Could you check a few things on this model? Use its own coordinates, in mm. Face numbers are marked on the shaded views. A direction names the side the tool comes from. Coordinates: 2 decimals unless noted, no trailing zeros. Order: outer loops, then holes, each group sorted by start corner. A loop starts at its lowest first (then second) coordinate and runs counter-clockwise, first axis right, second up. Notation, with made-up numbers: (-15.75, -1) -> (37.25, -1) arc R31 cw to (37.25, 26) -> close; hole circle Ø3 at (-38, 25.25). An arc over 180 degrees is marked (long way). Put each result on its own line as item: value. Start each with the question number.
Q1. If we section it at D-D (y = 30.5): Please give me the cut outline in (x, z).
Q2. We'd pull the mould along X, two halves only. Please class the marked faces 1, 2 and 3: +X half, -X half, draft (parallel to the pull), parting line (faces both ways), or undercut.
Q3. If we section it at B-B (y = 6): Please give me the cut outline in (x, z).
Q4. Please list where these lines run through material, in increasing order: line 1 along Z through (x, y) = (9, 22.5); line 2 along Y through (x, z) = (-1.5, 10.75); line 3 along X through (y, z) = (25.5, -3.25).
Q5. Will these pins go through, and if not, where does the flat tip stop? pin 1 (5 mm diameter, centred on x = -5.5, z = 4, fed in from +Y); pin 2 (11 mm diameter, centred on y = 20, z = -2.5, fed in from -X); pin 3 (3.5 mm diameter, centred on y = 30.5, z = -13, fed in from -X).
Q6. For the marked faces 4, 5 and 6, which set-ups out of +Z, -Z, +X, -X, +Y, -Y let a thin tool reach every point of the face, with its end or its side?
Q7. If we section it at A-A (z = 0): Please give me the cut outline in (x, y).
Q8. If we section it at C-C (x = 6.5): Please give me the cut outline in (y, z), and give its area (3 significant figures).
from build123d import *

# Parameters (mm, degrees)
SKETCH1_W               = 35
SKETCH1_H               = 28
BOSS_EXTRUDE1_DEPTH     = 35
SKETCH2_W               = 33.80681128
SKETCH2_H               = 22
CUT_EXTRUDE1_DEPTH      = 31
CUT_EXTRUDE2_DEPTH      = 49.117044797
CUT_EXTRUDE2_DEPTH_BACK = 49.117044797
CUT_EXTRUDE3_REACH      = 40.252
CUT_EXTRUDE4_REACH      = 43.343


with BuildPart() as part:
    # Sketch1 → Boss-Extrude1 (new body)
    with BuildSketch(Plane(origin=(0, 0, 0), x_dir=(1, 0, 0), z_dir=(0, 1, 0))):
        Rectangle(SKETCH1_W, SKETCH1_H)
    extrude(amount=BOSS_EXTRUDE1_DEPTH)

    # Sketch2 → Cut-Extrude1 (cut)
    with BuildSketch(Plane(origin=(0, 35, 0), x_dir=(1, 0, 0), z_dir=(0, 1, 0))):
        with Locations((-3.40340564, 0)):
            Rectangle(SKETCH2_W, SKETCH2_H)
    extrude(amount=-CUT_EXTRUDE1_DEPTH, mode=Mode.SUBTRACT)

    # Sketch3 → Cut-Extrude2 (cut, two sides: drawn at the far end of the back side and taken through both)
    with BuildSketch(Plane.XY.offset(14).offset(-CUT_EXTRUDE2_DEPTH_BACK)):
        Polygon((9.5, 133.408144421), (9.5, 35), (9.5, 28.634736483), (-11.134736483, 8), (-17.5, 8), (-115.908144421, 8), (-255.07827691, 147.170132488), (-129.670132488, 272.57827691), align=None)
    extrude(amount=CUT_EXTRUDE2_DEPTH + CUT_EXTRUDE2_DEPTH_BACK, mode=Mode.SUBTRACT)

    # Sketch4 → Cut-Extrude3 (cut, up to next)
    with BuildSketch(Plane(origin=(0, 4, 0), x_dir=(1, 0, 0), z_dir=(0, 1, 0)), mode=Mode.PRIVATE) as cut_extrude3_sk1:
        with BuildLine():
            Line((4.5, -3.2), (-10.5, -3.2))
            ThreePointArc((-10.5, -3.2), (-13.7, 0), (-10.5, 3.2))
            Line((-10.5, 3.2), (4.5, 3.2))
            ThreePointArc((4.5, 3.2), (7.7, 0), (4.5, -3.2))
        make_face()
    cut_extrude3_tool1 = extrude(cut_extrude3_sk1.sketch, amount=-CUT_EXTRUDE3_REACH, mode=Mode.PRIVATE) & part.part
    add(cut_extrude3_tool1.solids().sort_by_distance((-3, 4, 0))[0], mode=Mode.SUBTRACT)

    # Sketch5 → Cut-Extrude4 (cut, up to next)
    with BuildSketch(Plane(origin=(13.5, 23.5, 0), x_dir=(0, 1, 0), z_dir=(-1, 0, 0)), mode=Mode.PRIVATE) as cut_extrude4_sk1:
        with BuildLine():
            Line((4.5, -3.2), (-10.5, -3.2))
            ThreePointArc((-10.5, -3.2), (-13.7, 0), (-10.5, 3.2))
            Line((-10.5, 3.2), (4.5, 3.2))
            ThreePointArc((4.5, 3.2), (7.7, 0), (4.5, -3.2))
        make_face()
    cut_extrude4_tool1 = extrude(cut_extrude4_sk1.sketch, amount=-CUT_EXTRUDE4_REACH, mode=Mode.PRIVATE) & part.part
    add(cut_extrude4_tool1.solids().sort_by_distance((13.5, 20.5, 0))[0], mode=Mode.SUBTRACT)


solid = part.part
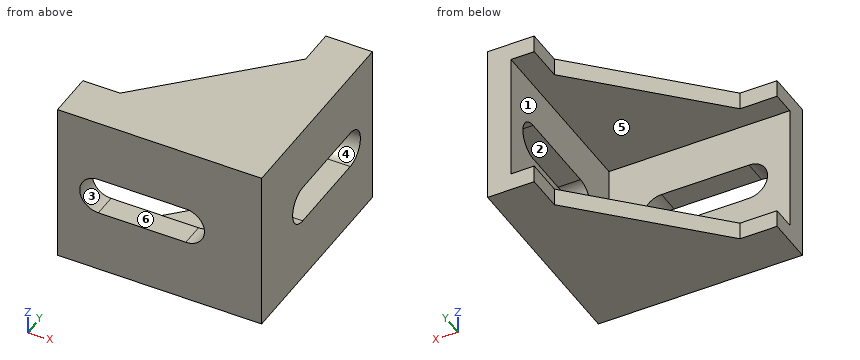
The answers:
1. outline: (9.5, -14) -> (17.5, -14) -> (17.5, -2) -> (13.5, -2) -> (13.5, -11) -> (9.5, -11) -> close; (9.5, 11) -> (13.5, 11) -> (13.5, 2) -> (17.5, 2) -> (17.5, 14) -> (9.5, 14) -> close
2. face 1: -X half
2. face 2: draft
2. face 3: undercut
3. outline: (-17.5, -14) -> (17.5, -14) -> (17.5, 14) -> (-17.5, 14) -> (-17.5, 11) -> (13.5, 11) -> (13.5, -11) -> (-17.5, -11) -> close
4. line 1: -14 to -11, 11 to 14
4. line 2: 0 to 4
4. line 3: 13.5 to 17.5
5. pin 1: y = 4
5. pin 2: x = 13.5
5. pin 3: x = 9.5
6. face 4: +X, -X
6. face 5: -X, +Y
6. face 6: +Y, -Y
7. outline: (-17.5, 0) -> (-13.7, 0) -> (-13.7, 4) -> (-17.5, 4) -> close; (7.7, 0) -> (17.5, 0) -> (17.5, 9.8) -> (13.5, 9.8) -> (13.5, 4) -> (7.7, 4) -> close; (13.5, 31.2) -> (17.5, 31.2) -> (17.5, 35) -> (13.5, 35) -> close
8. outline: (0, -14) -> (25.63, -14) -> (25.63, -11) -> (4, -11) -> (4, -2.5) -> (0, -2.5) -> close; (0, 2.5) -> (4, 2.5) -> (4, 11) -> (25.63, 11) -> (25.63, 14) -> (0, 14) -> close
8. area: 222 mm^2
